Source: CAD feature listing. Evaluate the final solid. Frame: model axes, mm. A direction names the side the tool comes from. Give positions to 0.01 mm unless a question says otherwise; leave off trailing zeros. Write each loop counter-clockwise with the first axis right and the second up, starting at its lowest first coordinate (ties: lowest second). Pieces come first, ordered by that corner, then holes. Notation, with made-up numbers: M -33,-13.75 L -12,-13.75 A18 cw -12,-7.75 Z; hole C 37,51 d2. An arc over 180 degrees is marked long. Use CSV: the item, a comma, the result in double quotes. Start each with the question number.
Autodesk Fusion 360 part; units mm, degrees
sketch "Sketch1" plane through (0, 0, 0) normal (0, 1, 0) x (1, 0, 0)
  line L0 (0, 0) -> (-100, 0) construction
  line L1 (-100, 0) -> (-100, -100) construction
  line L2 (-100, -100) -> (0, -100) construction
  line L3 (0, -100) -> (0, 0) construction
  line L4 (10, 20) -> (-110, 20)
  line L5 (-120, 10) -> (-120, -110)
  line L6 (-110, -120) -> (10, -120)
  line L7 (20, -110) -> (20, 10)
  circle A0 centre (0, 0) radius 1.65
  circle A1 centre (-100, 0) radius 1.65
  circle A2 centre (0, -100) radius 1.65
  circle A3 centre (-100, -100) radius 1.65
  arc A4 (10, -120) -> (20, -110) centre (10, -110) ccw
  arc A5 (-120, -110) -> (-110, -120) centre (-110, -110) ccw
  arc A6 (-110, 20) -> (-120, 10) centre (-110, 10) ccw
  arc A7 (20, 10) -> (10, 20) centre (10, 10) ccw
  dimension "d1" = 100
  dimension "d2" = 100
  dimension "d4" = 3.3
  dimension "d7" = -100
  dimension "d8" = -100
  dimension "d9" = 10
extrude "Extrude1" add sketch "Sketch1" along normal blind 7 makes body 1
sketch "Sketch2" plane through (0, 7, 0) normal (0, 1, 0) x (-1, 0, 0)
  circle A0 centre (0, 0) radius 1.65
  circle A1 centre (100, 100) radius 1.65
  circle A2 centre (0, 100) radius 1.65
  circle A3 centre (100, 0) radius 1.65
  arc A4 (-20, -10) -> (-10, -20) centre (-10, -10) ccw
  line L0 (-10, -20) -> (110, -20)
  arc A5 (110, -20) -> (120, -10) centre (110, -10) ccw
  line L1 (120, -10) -> (120, 110)
  arc A6 (120, 110) -> (110, 120) centre (110, 110) ccw
  line L2 (110, 120) -> (-10, 120)
  arc A7 (-10, 120) -> (-20, 110) centre (-10, 110) ccw
  line L3 (-20, 110) -> (-20, -10)
  circle A8 centre (0, 0) radius 2.8
  circle A9 centre (100, 0) radius 2.8
  circle A10 centre (0, 100) radius 2.8
  circle A11 centre (100, 100) radius 2.8
  dimension "d12" = 5.6
  dimension "d15" = 100
  dimension "d16" = 100
extrude "Extrude2" cut sketch "Sketch2" against normal blind 3 contours A8 | A9 | A10 | A11 bodies 1
sketch "Sketch3" plane through (0, 0, 0) normal (0, 1, 0) x (1, 0, 0)
  line L0 (-1, 0) -> (-19, 0)
  line L1 (0, -19) -> (0, -1)
  line L2 (-1, -20) -> (-2.5858, -20)
  line L3 (-20, -1) -> (-20, -2.5858)
  line L4 (-19.7071, -3.2929) -> (-3.2929, -19.7071)
  line L5 (-14.4645, -5.7071) -> (-5.7071, -14.4645)
  line L6 (-5, -4) -> (-13.7574, -4)
  line L7 (-4, -13.7574) -> (-4, -5)
  arc A0 (-1, -20) -> (0, -19) centre (-1, -19) ccw
  arc A1 (-3.2929, -19.7071) -> (-2.5858, -20) centre (-2.5858, -19) ccw
  arc A2 (0, -1) -> (-1, 0) centre (-1, -1) ccw
  arc A3 (-19, 0) -> (-20, -1) centre (-19, -1) ccw
  arc A4 (-20, -2.5858) -> (-19.7071, -3.2929) centre (-19, -2.5858) ccw
  arc A5 (-5.7071, -14.4645) -> (-4, -13.7574) centre (-5, -13.7574) ccw
  arc A6 (-4, -5) -> (-5, -4) centre (-5, -5) ccw
  arc A7 (-13.7574, -4) -> (-14.4645, -5.7071) centre (-13.7574, -5) ccw
  point P0 (-20, 0)
  point P1 (0, -20)
  point P2 (-3, -20)
  point P3 (-20, -3)
  dimension "d19" = 20
  dimension "d20" = 20
  dimension "d23" = 3
  dimension "d24" = 3
  dimension "d26" = 1
  dimension "d27" = 1
  dimension "d30" = 2
extrude "Extrude3" add sketch "Sketch3" along normal blind 20 separate body makes body 2
sketch "Sketch4" plane through (0, 0, 0) normal (0, 0, -1) x (-1, 0, 0)
  line L0 (1, 0) -> (19, 0)
  line L1 (19, 0) -> (19, 20)
  line L2 (19, 20) -> (1, 20)
  line L3 (1, 20) -> (1, 0)
  circle A0 centre (10, 10) radius 1.65
  dimension "d31" = 3.3
extrude "Extrude5" cut sketch "Sketch4" against normal blind 30 contours A0 bodies 2
sketch "Sketch5" plane through (0, 0, 0) normal (1, 0, 0) x (0, 0, -1)
  line L0 (-19, 0) -> (-1, 0)
  line L1 (-1, 0) -> (-1, 20)
  line L2 (-1, 20) -> (-19, 20)
  line L3 (-19, 20) -> (-19, 0)
  circle A0 centre (-10, 10) radius 1.65
  dimension "d34" = 3.3
extrude "Extrude6" cut sketch "Sketch5" against normal blind 49 contours A0 bodies 2
sketch "Sketch6" plane through (-11.5, 0, 11.5) normal (-0.7071, 0, 0.7071) x (0.7071, 0, 0.7071)
  line L0 (-11.6066, 0) -> (11.6066, 0)
  line L1 (11.6066, 0) -> (11.6066, 20)
  line L2 (11.6066, 20) -> (-11.6066, 20)
  line L3 (-11.6066, 20) -> (-11.6066, 0)
  ellipse E0 centre (-2.1213, 10) end of major axis (-4.4548, 10) minor radius 1.65 (0, 10.6874) -> (0, 9.3126) ccw
  ellipse E1 centre (2.1213, 10) end of major axis (-0.2121, 10) minor radius 1.65 (0, 9.3126) -> (0, 10.6874) ccw
  circle A0 centre (0, 10) radius 6
  dimension "d37" = 12
extrude "Extrude7" cut sketch "Sketch6" against normal blind 3 contours E0 E1 | A0 bodies 2
extrude "Extrude4" [suppressed]
hidden bodies 1
Item 1: Section A-A (y = 18). Return the cut outline in (x, z), plus the area to 3 significant figures.
Item 2: Material intervals for probe 1 along Y at (x, z) = (-1.85, 10); probe 2 along X at (y, z) = (1.75, 18); probe 3 along Z at (x, y) = (-12.75, 12.25), sorted ascending.
Item 3: Contact query for flat-ended pins moving along their axis: pin 1 Ø6 at (y, z) = (4.5, 13) entering from +X; pin 2 Ø7 at (x, y) = (-11, 6) entering from +Z; pin 3 Ø1 at (x, y) = (-5, 7) entering from +Z; pin 4 Ø9.5 at (y, z) = (13.5, 10) entering from -X. Output: stop coordinate, or through.
Item 4: Section D-D (y = 9.5). Return the cut outline in (x, z).
Item 5: Set-up query: faces 1 (the flat face through (-8, 20, 3)), 2 (the cylindrical face through (-4.301, 9.86, 4.285)). Return all of +Z, -Z, +X, -X, +Y, -Y with unobstructed straight access to the full face (end or side cutting, diameter ignored); none if empty.
Item 6: Pull-direction query (X, two-part tool) for faces 3 (the cylindrical face through (-0.285, 9.86, 19.699)), 4 (the flat face through (-12, 10, 0)), 5 (the flat face through (-20, 10, 2)), 6 (the cylindrical face through (-14.687, 9.86, 4.633)); classes: released by +X, released by -X, zero draft, split by the parting line, or undercut.
Item 7: Section B-B (y = 6.75). Return the cut outline in (x, z).
Item 8: Section C-C (x = -10). State how many separate pieces and enclosed holes the cut face has, plus the area to 3 significant figures.
Output values:
1,outline,"M -20,1 A1 ccw -19,0 L -1,0 A1 ccw 0,1 L 0,19 A1 ccw -1,20 L -2.59,20 A1 ccw -3.29,19.71 L -19.71,3.29 A1 ccw -20,2.59 Z; hole M -14.46,5.71 A1 ccw -13.76,4 L -5,4 A1 ccw -4,5 L -4,13.76 A1 ccw -5.71,14.46 Z"
1,area,"183 mm2"
2,probe 1,"y = 0 to 8.35, 11.65 to 20"
2,probe 2,"x = -5 to 0"
2,probe 3,"z = 0 to 4"
3,pin 1,"stops at x = 0"
3,pin 2,"stops at z = 15.5"
3,pin 3,"stops at z = 18.5"
3,pin 4,"stops at x = -17.75"
4,outline,"M -20,1 A1 ccw -19,0 L -11.57,0 L -11.57,4 L -13.76,4 A1 cw -14.46,5.71 L -14.31,5.86 L -15.73,7.27 L -19.71,3.29 A1 ccw -20,2.59 Z; M -8.43,0 L -1,0 A1 ccw 0,1 L 0,8.43 L -4,8.43 L -4,5 A1 cw -5,4 L -8.43,4 Z; M -7.27,15.73 L -5.86,14.31 L -5.71,14.46 A1 cw -4,13.76 L -4,11.57 L 0,11.57 L 0,19 A1 ccw -1,20 L -2.59,20 A1 ccw -3.29,19.71 Z"
5,face 1,"+Z, -Z, +X, -X, +Y"
5,face 2,"+Y, -Y"
6,face 3,"released by +X"
6,face 4,"zero draft"
6,face 5,"released by -X"
6,face 6,"undercut"
7,outline,"M -20,1 A1 ccw -19,0 L -1,0 A1 ccw 0,1 L 0,19 A1 ccw -1,20 L -2.59,20 A1 ccw -3.29,19.71 L -7.93,15.07 L -6.52,13.65 L -5.71,14.46 A1 cw -4,13.76 L -4,5 A1 cw -5,4 L -13.76,4 A1 cw -14.46,5.71 L -13.65,6.52 L -15.07,7.93 L -19.71,3.29 A1 ccw -20,2.59 Z"
8,separate pieces,"4"
8,enclosed holes,"0"
8,area,"90.2 mm2"
